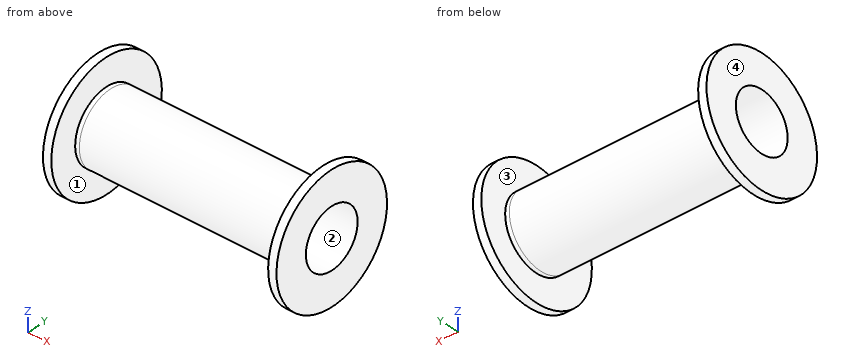
```python
from build123d import *

# Parameters (mm, degrees)
ESBO_O2_R             = 14.95
ESBO_O2_R_2           = 8.5
CORTE_EXTRUS_O1_DEPTH = 1
ESBO_O3_R             = 14.95
ESBO_O3_R_2           = 8.5
CORTE_EXTRUS_O2_DEPTH = 1


with BuildPart() as part:
    # Esboço1 → Revolução1 (revolve)
    with BuildSketch(Plane(origin=(0, 0, 0), x_dir=(1, 0, 0), z_dir=(0, 1, 0))):
        Polygon((-56, -7), (-56, -14.95), (-53, -14.95), (-53, -8.5), (-3, -8.5), (-3, -14.95), (0, -14.95), (0, -7), align=None)
    revolve(axis=Axis((-102.959505757, 0, 0), (1, 0, 0)))

    # Esboço2 → Corte-extrusão1 (cut)
    with BuildSketch(Plane(origin=(-53, 0, 0), x_dir=(0, 0, -1), z_dir=(1, 0, 0))):
        Circle(ESBO_O2_R)
        Circle(ESBO_O2_R_2, mode=Mode.SUBTRACT)
    extrude(amount=-CORTE_EXTRUS_O1_DEPTH, mode=Mode.SUBTRACT)

    # Esboço3 → Corte-extrusão2 (cut)
    with BuildSketch(Plane.ZY.offset(3)):
        Circle(ESBO_O3_R)
        Circle(ESBO_O3_R_2, mode=Mode.SUBTRACT)
    extrude(amount=-CORTE_EXTRUS_O2_DEPTH, mode=Mode.SUBTRACT)


solid = part.part
```
The listing builds one solid part. Answer for the finished solid, in the listing's coordinates (mm). Face numbers are marked on the shaded views. A direction names the side the tool comes from. Coordinates: 2 decimals unless noted, no trailing zeros. Write each loop counter-clockwise with the first axis right and the second up, starting at its lowest first coordinate (ties: lowest second). Pieces come first, ordered by that corner, then holes. Notation, with made-up numbers: (20, -16) - (75, -16) arc R4 ccw to (75, -11) - close; hole circle Ø3 at (56, -9.5). An arc over 180 degrees is marked (long way). Return JSON: item names as keys, results as strings. Group by question number.
1. A cutting plane is placed at A-A, the plane y = 0. Determine the outline of the cut face in (x, z).
2. Which of the six approach directions +Z, -Z, +X, -X, +Y, -Y give full straight-line access (tool end or side, diameter ignored) to the marked faces 3 and 4?
3. A cutting plane is placed at D-D, the plane y = 12. Determine the outline of the cut face in (x, z), plus the area to 3 significant figures.
4. Determine the mould class of the marked faces 1 and 2 for opening direction Z: released by +Z, released by -Z, zero draft, split by the parting line, or undercut.
5. A cutting plane is placed at C-C, the plane x = -16.5. Determine the outline of the cut face in (y, z).
6. Given pin 1 (5 mm diameter, centred on x = -31, z = 7, fed in from +Y); pin 2 (2 mm diameter, centred on x = -33, y = -6, fed in from +Z); pin 3 (1 mm diameter, centred on x = -17.5, z = -8, fed in from -Y); pin 4 (12.5 mm diameter, centred on y = 0, z = 0, fed in from -X), each flat-ended and moving along its own axis, determine where each tip first touches the part or whether it passes through.
7. Straight lines are drawn through the part: L1, parallel to X at y = 9.5, z = 9; L2, parallel to Y at x = -42, z = 0. For each, find the intervals that lie inside material, in ascending order.
Ans:
{
 "1": {"outline": "(-56, -14.95) - (-54, -14.95) - (-54, -8.5) - (-2, -8.5) - (-2, -14.95) - (0, -14.95) - (0, -7) - (-56, -7) - close; (-56, 7) - (0, 7) - (0, 14.95) - (-2, 14.95) - (-2, 8.5) - (-54, 8.5) - (-54, 14.95) - (-56, 14.95) - close"},
 "2": {"face 3": "none", "face 4": "+Z, -Z, -X, +Y, -Y"},
 "3": {"outline": "(-56, -8.92) - (-54, -8.92) - (-54, 8.92) - (-56, 8.92) - close; (-2, -8.92) - (0, -8.92) - (0, 8.92) - (-2, 8.92) - close", "area": "71.3 mm²"},
 "4": {"face 1": "zero draft", "face 2": "undercut"},
 "5": {"outline": "circle Ø17 at (0, 0); hole circle Ø14 at (0, 0)"},
 "6": {"pin 1": "y = 7.21", "pin 2": "z = 6.87", "pin 3": "y = -4", "pin 4": "through"},
 "7": {"L1": "-56 to -54, -2 to 0", "L2": "-8.5 to -7, 7 to 8.5"}
}
